```python
from build123d import *

# Parameters (mm, degrees)
F0_W     = 28
F0_H     = 28
F1_DEPTH = 24
F2_W     = 10
F2_H     = 10
F2_W_2   = 12
F2_H_2   = 12
F3_DEPTH = 8
F4_W     = 12
F4_H     = 12
F4_W_2   = 10
F4_H_2   = 10
F5_DEPTH = 8


with BuildPart() as f1:
    # F0 (on Top) → F1 (new body)
    with BuildSketch(Plane.XY):
        with Locations((-14, -14)):
            Rectangle(F0_W, F0_H)
        with Locations((14, -14)):
            Rectangle(F0_W, F0_H)
        with Locations((14, 14)):
            Rectangle(F0_W, F0_H)
        with Locations((-14, 14)):
            Rectangle(F0_W, F0_H)
    extrude(amount=F1_DEPTH)

    # F2 (on face) → F3 (join)
    with BuildSketch(Plane(origin=(0, 28, 0), x_dir=(-1, 0, 0), z_dir=(0, 1, 0))):
        with Locations((-16.822546, 8.821471)):
            Rectangle(F2_W, F2_H)
        with Locations((16.008998, 9.988178)):
            Rectangle(F2_W_2, F2_H_2)
    extrude(amount=F3_DEPTH)

    # F4 (on face) → F5 (join)
    with BuildSketch(Plane.XZ.offset(28)):
        with Locations((-18.081427, 12.249541)):
            Rectangle(F4_W, F4_H)
        with Locations((17.498491, 11.249541)):
            Rectangle(F4_W_2, F4_H_2)
    extrude(amount=F5_DEPTH)


solid = f1.part
```
Could you check a few things on this model? Use its own coordinates, in mm. A direction names the side the tool comes from. Coordinates: 2 decimals unless noted, no trailing zeros. Write each loop counter-clockwise with the first axis right and the second up, starting at its lowest first coordinate (ties: lowest second). Pieces come first, ordered by that corner, then holes. Notation, with made-up numbers: (48, -9.5) -> (107, -9.5) arc R37 ccw to (107, 28.5) -> close; hole circle Ø4 at (11.25, 63). An arc over 180 degrees is marked (long way). Return JSON: item names as keys, results as strings.
(1) Which directions (+Z, -Z, +X, -X, +Y, -Y) give clear straight access to the entire face, cutting with the end or side of a thin tool? Please do faces 1 (the flat face through (21.823, 32, 9)), 2 (the flat face through (-16, 32, 3.988)), 3 (the flat face through (17, -32, 6.25)), 4 (the flat face through (-10.009, 32, 10)), 5 (the flat face through (12.498, -32, 11)).
Numbers:
{"face 1": "+Z, -Z, +X, +Y", "face 2": "-Z, -X, +Y", "face 3": "-Z, +X, -X, -Y", "face 4": "+Z, -Z, +Y", "face 5": "+Z, -Z, -Y"}
(2) Imagine slicing it at A-A, the plane z = 9.75. Please give me the cut outline in (x, y), then the cut area to 3 significant figures.
Numbers:
{"outline": "(-28, -28) -> (-24.08, -28) -> (-24.08, -36) -> (-12.08, -36) -> (-12.08, -28) -> (12.5, -28) -> (12.5, -36) -> (22.5, -36) -> (22.5, -28) -> (28, -28) -> (28, 28) -> (21.82, 28) -> (21.82, 36) -> (11.82, 36) -> (11.82, 28) -> (-10.01, 28) -> (-10.01, 36) -> (-22.01, 36) -> (-22.01, 28) -> (-28, 28) -> close", "area": "3,490 mm2"}
(3) Imagine slicing it at C-C, the plane z = 3. Please give me the cut outline in (x, y).
Numbers:
{"outline": "(-28, -28) -> (28, -28) -> (28, 28) -> (-28, 28) -> close"}
(4) I need wall thicknesses on L1, parallel to Y at x = 26, z = 7.25; L2, parallel to Y at x = -12.5, z = 17; L3, parallel to Z at x = -14, y = -30.5. Which ranges of each line are inside material? Lowest first, please.
Numbers:
{"L1": "y = -28 to 28", "L2": "y = -36 to 28", "L3": "z = 6.25 to 18.25"}
(5) Imagine slicing it at D-D, the plane x = 6. Please give me the cut outline in (y, z), then the cut area to 3 significant figures.
Numbers:
{"outline": "(-28, 0) -> (28, 0) -> (28, 24) -> (-28, 24) -> close", "area": "1,340 mm2"}
(6) I'm going to push flat-ended pins straight in: pin 1 (2.5 mm diameter, centred on y = 34, z = 11, fed in from -X); pin 2 (4 mm diameter, centred on x = 15.5, y = -32, fed in from +Z); pin 3 (4 mm diameter, centred on x = -15.5, y = 31.5, fed in from +Z); pin 4 (12 mm diameter, centred on x = 3.5, y = 19, fed in from -Z). Where does each tip first touch, or does it pass through?
Numbers:
{"pin 1": "stops at x = -22.01", "pin 2": "stops at z = 16.25", "pin 3": "stops at z = 15.99", "pin 4": "stops at z = 0"}
(7) We'd pull the mould along X, two halves only. Please class faces 6 (the flat face through (0, -28, 12)), 7 (the flat face through (28, 0, 12)), 8 (the flat face through (-16, 32, 15.988)): +X half, -X half, draft (parallel to the pull), parting line (faces both ways), or undercut.
Numbers:
{"face 6": "undercut", "face 7": "+X half", "face 8": "draft"}
(8) Imagine slicing it at B-B, the plane x = -20. Please give me the cut outline in (y, z), then the cut area to 3 significant figures.
Numbers:
{"outline": "(-36, 6.25) -> (-28, 6.25) -> (-28, 0) -> (28, 0) -> (28, 3.99) -> (36, 3.99) -> (36, 15.99) -> (28, 15.99) -> (28, 24) -> (-28, 24) -> (-28, 18.25) -> (-36, 18.25) -> close", "area": "1,540 mm2"}
